Source: CAD feature listing. Evaluate the final solid. Frame: model axes, mm. Face numbers are marked on the shaded views. Give positions to 0.01 mm unless a question says otherwise; leave off trailing zeros. Order: outer loops, then holes, each group sorted by start corner. A loop starts at its lowest first (then second) coordinate and runs counter-clockwise, first axis right, second up. Notation, with made-up numbers: M 76.5,67 L 82.5,67 A26 cw 82.5,90 Z; hole C 61.5,64 d2. An arc over 180 degrees is marked long. One line per question, with ' | ' between items. Start each with the question number.
from build123d import *

# Parameters (mm, degrees)
F0_W      = 85
F0_H      = 23
F0_H_2    = 40
F1_DEPTH  = 3
F2_W      = 3
F2_H      = 23
F3_DEPTH  = 24
F4_W      = 3
F4_H      = 23
F5_DEPTH  = 25
F6_R      = 4
F7_DEPTH  = 200
F8_R      = 2
F9_DEPTH  = 250
F11_DEPTH = 250


with BuildPart() as f1:
    # F0 (on Top) → F1 (new body)
    with BuildSketch(Plane.XY):
        with Locations((42.5, 11.5)):
            Rectangle(F0_W, F0_H)
        with Locations((42.5, -20)):
            Rectangle(F0_W, F0_H_2)
    extrude(amount=F1_DEPTH)

    # F2 (on face) → F3 (join)
    with BuildSketch(Plane.XY.offset(3)):
        with Locations((1.5, 11.5)):
            Rectangle(F2_W, F2_H)
        with Locations((83.5, 11.5)):
            Rectangle(F2_W, F2_H)
    extrude(amount=F3_DEPTH)

    # F4 (on face) → F5 (join)
    with BuildSketch(Plane.XY.offset(27)):
        with Locations((1.5, 11.5)):
            Rectangle(F4_W, F4_H)
    extrude(amount=F5_DEPTH)

    # F6 (on face) → F7 (cut)
    with BuildSketch(Plane.YZ.offset(85)):
        with Locations((11.5, 13.5)):
            Circle(F6_R)
    extrude(amount=-F7_DEPTH, mode=Mode.SUBTRACT)

    # F8 (on face) → F9 (cut)
    with BuildSketch(Plane(origin=(0, 0, 0), x_dir=(0, -1, 0), z_dir=(-1, 0, 0))):
        with BuildLine():
            ThreePointArc((-1.5, 13.5), (-3.5, 15.5), (-5.5, 13.5))
            ThreePointArc((-5.5, 13.5), (-3.5, 11.5), (-1.5, 13.5))
        make_face()
        with Locations((-19.5, 13.5)):
            Circle(F8_R)
    extrude(amount=-F9_DEPTH, mode=Mode.SUBTRACT)

    # F10 (on face) → F11 (cut)
    with BuildSketch(Plane.YZ.offset(85)):
        with BuildLine():
            ThreePointArc((13.5, 21.5), (10.085786, 22.914214), (11.5, 19.5))
            ThreePointArc((11.5, 19.5), (12.914214, 20.085786), (13.5, 21.5))
        make_face()
        with BuildLine():
            ThreePointArc((13.5, 5.5), (12.914214, 6.914214), (11.5, 7.5))
            ThreePointArc((11.5, 7.5), (10.085786, 4.085786), (13.5, 5.5))
        make_face()
    extrude(amount=-F11_DEPTH, mode=Mode.SUBTRACT)


solid = f1.part
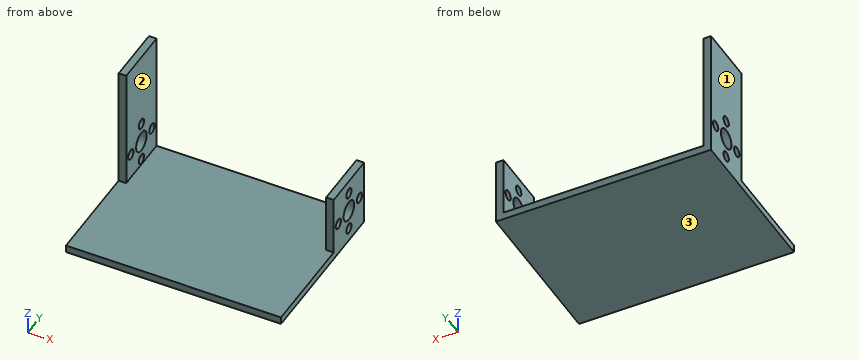
Item 1: Cut plane D-D on z = 47. Return the cut outline in (x, y), and give its area (3 significant figures).
Item 2: Line query: line 1 (Z direction, x = 83.9, y = 11.5); line 2 (Y direction, x = 84, z = 21.5); line 3 (Z direction, x = 67, y = 15). Output: solid intervals per line, ascending.
Item 3: Cut plane A-A on y = 3.5. Return the cut outline in (x, z).
Item 4: Cut plane C-C on x = 22. Return the cut outline in (y, z), and give its area (3 significant figures).
Item 5: Pin query (flat end, axial travel): pin 1 Ø3 at (x, y) = (52, -14.5) entering from +Z; pin 2 Ø2.5 at (x, z) = (83, 12) entering from -Y; pin 3 Ø3.5 at (x, y) = (84, 10) entering from +Z. Return the tip coordinate at first contact, or that it passes through.
Item 6: Cut plane B-B on z = 25. Return the cut outline in (x, y).
Item 7: Mould query, pull axis X, two halves, no side actions, for the marked faces 1, 2 and 3. Classes: pulls with the +X half, pulls with the -X half, needs draft (parallel to the pull), parting line crosses it, or undercut.
Results are:
1) outline: M 0,0 L 3,0 L 3,23 L 0,23 Z | area: 69.0 mm2
2) line 1: z = 0 to 3.5, 7.5 to 9.5, 17.5 to 19.5, 23.5 to 27 | line 2: y = 0 to 9.5, 13.5 to 23 | line 3: z = 0 to 3
3) outline: M 0,0 L 85,0 L 85,11.5 L 82,11.5 L 82,3 L 3,3 L 3,11.5 L 0,11.5 Z; M 0,15.5 L 3,15.5 L 3,52 L 0,52 Z; M 82,15.5 L 85,15.5 L 85,27 L 82,27 Z
4) outline: M -40,0 L 23,0 L 23,3 L -40,3 Z | area: 189 mm2
5) pin 1: stops at z = 3 | pin 2: stops at y = 0 | pin 3: stops at z = 27
6) outline: M 0,0 L 3,0 L 3,23 L 0,23 Z; M 82,0 L 85,0 L 85,23 L 82,23 Z
7) face 1: pulls with the -X half | face 2: undercut | face 3: needs draft
